The model under review builds one solid part; all positions refer to its coordinate system, in mm. A direction names the side the tool comes from. Round coordinates to 2 decimals unless told otherwise and drop trailing zeros. Order: outer loops, then holes, each group sorted by start corner. A loop starts at its lowest first (then second) coordinate and runs counter-clockwise, first axis right, second up.
from build123d import *

# Parameters (mm, degrees)
BOSS_EXTRUDE1_DEPTH = 56.75
SKETCH2_W           = 5
SKETCH2_H           = 85
SKETCH2_R           = 1.5
CUT_EXTRUDE1_DEPTH  = 2
SKETCH3_R           = 6.35
SKETCH3_R_2         = 1.5
CUT_EXTRUDE2_DEPTH  = 3
CHAMFER1_SIZE       = 0.5
CUT_EXTRUDE3_DEPTH  = 5.5
CUT_EXTRUDE4_DEPTH  = 10


with BuildPart() as part:
    # Sketch1 → Boss-Extrude1 (new body, symmetric)
    with BuildSketch(Plane.XY):
        Polygon((0, 50), (0, -50), (7.5, -50), (7.5, -42.5), (2, -42.5), (2, 42.5), (7.5, 42.5), (7.5, 50), align=None)
    extrude(amount=BOSS_EXTRUDE1_DEPTH, both=True)

    # Sketch2 → Cut-Extrude1 (cut)
    with BuildSketch(Plane(origin=(2, 0, 0), x_dir=(0, 0, -1), z_dir=(1, 0, 0))):
        with Locations((-54.25, 0)):
            Rectangle(SKETCH2_W, SKETCH2_H)
        with Locations((54.25, 0)):
            Rectangle(SKETCH2_W, SKETCH2_H)
        with Locations((-47.75, 17.5)):
            Circle(SKETCH2_R)
        with Locations((-47.75, -17.5)):
            Circle(SKETCH2_R)
        with Locations((47.75, 17.5)):
            Circle(SKETCH2_R)
        with Locations((47.75, -17.5)):
            Circle(SKETCH2_R)
    extrude(amount=-CUT_EXTRUDE1_DEPTH, mode=Mode.SUBTRACT)

    # Sketch3 → Cut-Extrude2 (cut, through all)
    with BuildSketch(Plane(origin=(2, 0, 0), x_dir=(0, 0, -1), z_dir=(1, 0, 0))):
        Circle(SKETCH3_R)
        with Locations((39.75, 30.5)):
            Circle(SKETCH3_R_2)
        with Locations((39.75, -30.5)):
            Circle(SKETCH3_R_2)
        with BuildLine():
            Line((-29.899655804, -39.5), (29.899655804, -39.5))
            ThreePointArc((29.899655804, -39.5), (32.863003185, -37.464823364), (32.027336169, -33.968392001))
            Line((32.027336169, -33.968392001), (8.946350194, -13.129558949))
            ThreePointArc((8.946350194, -13.129558949), (7.399307524, -12.392275536), (5.701057458, -12.622220243))
            ThreePointArc((5.701057458, -12.622220243), (0, -13.85), (-5.701057458, -12.622220243))
            ThreePointArc((-5.701057458, -12.622220243), (-7.399307524, -12.392275536), (-8.946350194, -13.129558949))
            Line((-8.946350194, -13.129558949), (-32.027336169, -33.968392001))
            ThreePointArc((-32.027336169, -33.968392001), (-32.863003185, -37.464823364), (-29.899655804, -39.5))
        make_face()
        with BuildLine():
            Line((-43.75, -27.303546383), (-43.75, 27.303546383))
            ThreePointArc((-43.75, 27.303546383), (-41.864426198, 30.204926241), (-38.447319635, 29.660154382))
            Line((-38.447319635, 29.660154382), (-13.972366805, 7.562768399))
            ThreePointArc((-13.972366805, 7.562768399), (-13.081370721, 6.098851109), (-13.137175803, 4.386013216))
            ThreePointArc((-13.137175803, 4.386013216), (-13.85, 0), (-13.137175803, -4.386013216))
            ThreePointArc((-13.137175803, -4.386013216), (-13.081370721, -6.098851109), (-13.972366805, -7.562768399))
            Line((-13.972366805, -7.562768399), (-38.447319635, -29.660154382))
            ThreePointArc((-38.447319635, -29.660154382), (-41.864426198, -30.204926241), (-43.75, -27.303546383))
        make_face()
        with BuildLine():
            Line((-29.899655804, 39.5), (29.899655804, 39.5))
            ThreePointArc((29.899655804, 39.5), (32.863003185, 37.464823364), (32.027336169, 33.968392001))
            Line((32.027336169, 33.968392001), (8.946350194, 13.129558949))
            ThreePointArc((8.946350194, 13.129558949), (7.399307524, 12.392275536), (5.701057458, 12.622220243))
            ThreePointArc((5.701057458, 12.622220243), (0, 13.85), (-5.701057458, 12.622220243))
            ThreePointArc((-5.701057458, 12.622220243), (-7.399307524, 12.392275536), (-8.946350194, 13.129558949))
            Line((-8.946350194, 13.129558949), (-32.027336169, 33.968392001))
            ThreePointArc((-32.027336169, 33.968392001), (-32.863003185, 37.464823364), (-29.899655804, 39.5))
        make_face()
        with BuildLine():
            Line((43.75, -20.159375539), (43.75, 20.159375539))
            ThreePointArc((43.75, 20.159375539), (39.978852396, 25.962135255), (33.144639269, 24.872591538))
            Line((33.144639269, 24.872591538), (13.972366805, 7.562768399))
            ThreePointArc((13.972366805, 7.562768399), (13.081370721, 6.098851109), (13.137175803, 4.386013216))
            ThreePointArc((13.137175803, 4.386013216), (13.85, 0), (13.137175803, -4.386013216))
            ThreePointArc((13.137175803, -4.386013216), (13.081370721, -6.098851109), (13.972366805, -7.562768399))
            Line((13.972366805, -7.562768399), (33.144639269, -24.872591538))
            ThreePointArc((33.144639269, -24.872591538), (39.978852396, -25.962135255), (43.75, -20.159375539))
        make_face()
    extrude(amount=-CUT_EXTRUDE2_DEPTH, mode=Mode.SUBTRACT)

    # Chamfer1
    chamfer1_edges = [part.edges().sort_by_distance(p)[0] for p in [
        (0, -50, 0),
        (0, 50, 0),
    ]]
    chamfer(chamfer1_edges, length=CHAMFER1_SIZE)

    # Sketch4 → Cut-Extrude3 (cut)
    with BuildSketch(Plane(origin=(7.5, 0, 0), x_dir=(0, 0, -1), z_dir=(1, 0, 0))):
        with BuildLine():
            Line((43.575, -48), (-43.575, -48))
            ThreePointArc((-43.575, -48), (-45.82006403, -47.07006403), (-46.75, -44.825))
            Line((-46.75, -44.825), (-46.75, -43.5))
            ThreePointArc((-46.75, -43.5), (-47.042893219, -42.792893219), (-47.75, -42.5))
            Line((-47.75, -42.5), (47.75, -42.5))
            ThreePointArc((47.75, -42.5), (47.042893219, -42.792893219), (46.75, -43.5))
            Line((46.75, -43.5), (46.75, -44.825))
            ThreePointArc((46.75, -44.825), (45.82006403, -47.07006403), (43.575, -48))
        make_face()
        with BuildLine():
            Line((-46.75, 44.825), (-46.75, 43.5))
            ThreePointArc((-46.75, 43.5), (-47.042893219, 42.792893219), (-47.75, 42.5))
            Line((-47.75, 42.5), (47.75, 42.5))
            ThreePointArc((47.75, 42.5), (47.042893219, 42.792893219), (46.75, 43.5))
            Line((46.75, 43.5), (46.75, 44.825))
            ThreePointArc((46.75, 44.825), (45.82006403, 47.07006403), (43.575, 48))
            Line((43.575, 48), (-43.575, 48))
            ThreePointArc((-43.575, 48), (-45.82006403, 47.07006403), (-46.75, 44.825))
        make_face()
    extrude(amount=-CUT_EXTRUDE3_DEPTH, mode=Mode.SUBTRACT)

    # Sketch5 → Cut-Extrude4 (cut)
    with BuildSketch(Plane.ZY):
        with BuildLine():
            ThreePointArc((-51.75, 27.820508076), (-51.409258263, 30.408698527), (-50.410254038, 32.820508076))
            Line((-50.410254038, 32.820508076), (-48.285898385, 36.5))
            ThreePointArc((-48.285898385, 36.5), (-48.285898385, 40.5), (-51.75, 42.5))
            Line((-51.75, 42.5), (-51.75, 27.820508076))
        make_face()
        with BuildLine():
            ThreePointArc((-50.410254038, -32.820508076), (-51.409258263, -30.408698527), (-51.75, -27.820508076))
            Line((-51.75, -27.820508076), (-51.75, -42.5))
            ThreePointArc((-51.75, -42.5), (-48.285898385, -40.5), (-48.285898385, -36.5))
            Line((-48.285898385, -36.5), (-50.410254038, -32.820508076))
        make_face()
    cut_extrude4 = extrude(amount=-CUT_EXTRUDE4_DEPTH, mode=Mode.SUBTRACT)

    # Mirror1: Cut-Extrude4 across plane
    add(cut_extrude4.mirror(Plane.XY), mode=Mode.SUBTRACT)


solid = part.part
(1) Tool access review of faces 1 (the flat face through (1.014, 16.339, -23.693)), 2 (the cylindrical face through (4.79, -47.09, 45.8)), 3 (the flat face through (4, 42.5, -52)), 4 (the flat face through (4, 42.5, 52)): name each direction out of +Z, -Z, +X, -X, +Y, -Y from which nothing blocks a thin tool from reaching the whole face with its end or side.
(2) We need section A-A (y = 0). Give the boundary of the cut face in (x, z), and give its area (3 significant figures).
(3) Clearance check with flat-ended pins moving along their axes: P1, Ø2, axis at y = -34, z = -44.5, coming from the +X side; P2, Ø2, axis at x = 0.5, y = 5.5, coming from the -Z side. State where each tip first meets the part, or that it passes through.
(4) We need section B-B (z = 0). Give the boundary of the cut face in (x, y), and give its area (4 significant figures).
(5) We need section D-D (z = 17.5). Give the boundary of the cut face in (x, y).
(6) The part is to be moulded in two halves that separate along Y. For faces 5 (the cylindrical face through (1.01, 30.57, -38.25)), 6 (the flat face through (4, -46, -56.75)), 7 (the flat face through (4, -50, 1)), say which applies: pulls with the +Y half, pulls with the -Y half, needs draft (parallel to the pull), parting line crosses it, or undercut.
(7) To check wall thickness, follow L1, parallel to Y at x = 1.1, z = -39.75; L2, parallel to Y at x = 3.5, z = -49; L3, parallel to Y at x = 2.75, z = -7. State the ranges of each line that lie inside material, in increasing order.
(8) We need section C-C (y = 17.5). Give the boundary of the cut face in (x, z).
Verdict:
1. face 1: +X, -X
1. face 2: +X
1. face 3: -Z, +X
1. face 4: +Z, +X
2. outline: (0, -51.75) - (2, -51.75) - (2, -43.75) - (0, -43.75) - close; (0, -13.85) - (2, -13.85) - (2, -6.35) - (0, -6.35) - close; (0, 6.35) - (2, 6.35) - (2, 13.85) - (0, 13.85) - close; (0, 43.75) - (2, 43.75) - (2, 51.75) - (0, 51.75) - close
2. area: 62.0 mm2
3. P1: stops at x = 2
3. P2: stops at z = -51.75
4. outline: (0, -49.5) - (0.5, -50) - (7.5, -50) - (7.5, -48) - (2, -48) - (2, -39.5) - (0, -39.5) - close; (0, -13.85) - (2, -13.85) - (2, -6.35) - (0, -6.35) - close; (0, 6.35) - (2, 6.35) - (2, 13.85) - (0, 13.85) - close; (0, 39.5) - (2, 39.5) - (2, 48) - (7.5, 48) - (7.5, 50) - (0.5, 50) - (0, 49.5) - close
4. area: 93.75 mm2
5. outline: (0, -49.5) - (0.5, -50) - (7.5, -50) - (7.5, -48) - (2, -48) - (2, -39.5) - (0, -39.5) - close; (0, -20.85) - (2, -20.85) - (2, -10.75) - (0, -10.75) - close; (0, 10.75) - (2, 10.75) - (2, 20.85) - (0, 20.85) - close; (0, 39.5) - (2, 39.5) - (2, 48) - (7.5, 48) - (7.5, 50) - (0.5, 50) - (0, 49.5) - close
6. face 5: undercut
6. face 6: needs draft
6. face 7: pulls with the -Y half
7. L1: y = -50 to -32, -29 to -26.06, 26.06 to 29, 32 to 50
7. L2: y = -50 to -42.5, 42.5 to 50
7. L3: y = -50 to -48, 48 to 50
8. outline: (0, -51.75) - (2, -51.75) - (2, -49.25) - (0, -49.25) - close; (0, -46.25) - (2, -46.25) - (2, -43.75) - (0, -43.75) - close; (0, -24.98) - (2, -24.98) - (2, -13.79) - (0, -13.79) - close; (0, 13.79) - (2, 13.79) - (2, 24.98) - (0, 24.98) - close; (0, 43.75) - (2, 43.75) - (2, 46.25) - (0, 46.25) - close; (0, 49.25) - (2, 49.25) - (2, 51.75) - (0, 51.75) - close
